Model file for the job. Use its own axes, mm. Face numbers are marked on the shaded views. Give positions to 0.01 mm unless a question says otherwise; leave off trailing zeros. Write each loop counter-clockwise with the first axis right and the second up, starting at its lowest first coordinate (ties: lowest second). Pieces come first, ordered by that corner, then holes.
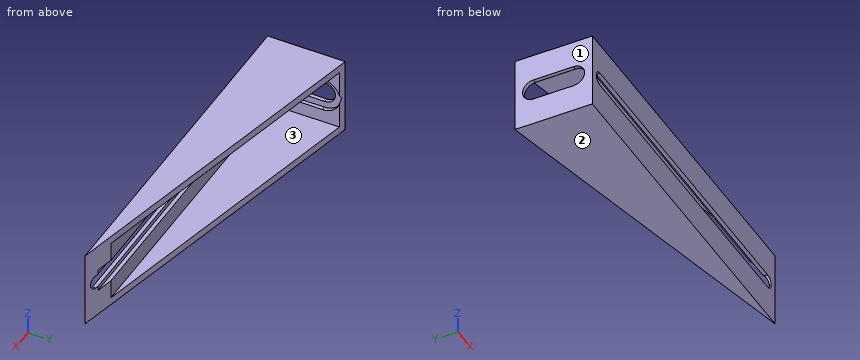
```python
from build123d import *

# Parameters (mm, degrees)
PAD_DEPTH            = 20
SKETCH001_W          = 88
SKETCH001_H          = 16
POCKET_DEPTH         = 18.001
POCKET001_DEPTH      = 2.001
POCKET002_DEPTH      = 1
POCKET002_DEPTH_BACK = -5
POCKET003_DEPTH      = 2.001
POCKET004_DEPTH      = 1


with BuildPart() as part:
    # Sketch → Pad (new body)
    with BuildSketch(Plane.XY):
        Polygon((0, 0), (0, 20), (90, 0), align=None)
    extrude(amount=PAD_DEPTH)

    # Sketch001 → Pocket (cut, through all)
    with BuildSketch(Plane.XZ.offset(-2)):
        with Locations((46, 10)):
            Rectangle(SKETCH001_W, SKETCH001_H)
    extrude(amount=-POCKET_DEPTH, mode=Mode.SUBTRACT)

    # Sketch002 (on Face9 of Pocket) → Pocket001 (cut, through all)
    with BuildSketch(Plane.YZ.offset(2)):
        with BuildLine():
            ThreePointArc((4.8, 12.8), (2, 10), (4.8, 7.2))
            Line((4.8, 7.2), (15.2, 7.2))
            ThreePointArc((15.2, 7.2), (18, 10), (15.2, 12.8))
            Line((4.8, 12.8), (15.2, 12.8))
        make_face()
    extrude(amount=-POCKET001_DEPTH, mode=Mode.SUBTRACT)

    # Sketch003 (on Face13 of Pocket001) → Pocket002 (cut, two sides)
    with BuildSketch(Plane.YZ.offset(2)) as pocket002_sk:
        with BuildLine():
            ThreePointArc((15.2, 5.5), (19.7, 10), (15.2, 14.5))
            Line((4.8, 14.5), (15.2, 14.5))
            ThreePointArc((4.8, 14.5), (3.317186, 14.248678), (2, 13.522783))
            Line((2, 13.522783), (2, 6.477217))
            ThreePointArc((2, 6.477217), (3.317186, 5.751322), (4.8, 5.5))
            Line((4.8, 5.5), (15.2, 5.5))
        make_face()
    extrude(amount=-POCKET002_DEPTH, mode=Mode.SUBTRACT)
    extrude(pocket002_sk.sketch, amount=-POCKET002_DEPTH_BACK, mode=Mode.SUBTRACT)

    # Sketch004 (on Face20 of Pocket002) → Pocket003 (cut, through all)
    with BuildSketch(Plane(origin=(0, 2, 0), x_dir=(-1, 0, 0), z_dir=(0, 1, 0))):
        with BuildLine():
            ThreePointArc((-86.2, 11.8), (-88, 10), (-86.2, 8.2))
            Line((-86.2, 8.2), (-3.8, 8.2))
            ThreePointArc((-3.8, 8.2), (-2, 10), (-3.8, 11.8))
            Line((-86.2, 11.8), (-3.8, 11.8))
        make_face()
    extrude(amount=-POCKET003_DEPTH, mode=Mode.SUBTRACT)

    # Sketch005 (on Face15 of Pocket003) → Pocket004 (cut)
    with BuildSketch(Plane(origin=(0, 2, 0), x_dir=(-1, 0, 0), z_dir=(0, 1, 0))):
        with BuildLine():
            ThreePointArc((-86.2, 13), (-89.2, 10), (-86.2, 7))
            Line((-86.2, 7), (-3.8, 7))
            ThreePointArc((-3.8, 7), (-2.851317, 7.15395), (-2, 7.6))
            Line((-2, 12.4), (-2, 7.6))
            ThreePointArc((-2, 12.4), (-2.851317, 12.84605), (-3.8, 13))
            Line((-86.2, 13), (-3.8, 13))
        make_face()
    extrude(amount=-POCKET004_DEPTH, mode=Mode.SUBTRACT)


solid = part.part
```
1. Slice it at C-C, the plane z = 3.5. Write the cut outline in (x, y).
Calculated:
outline: (0, 0) - (90, 0) - (81, 2) - (2, 2) - (2, 19.56) - (0, 20) - close
2. Slice it at B-B, the plane x = 54. Write the cut outline in (y, z), and give its area (3 significant figures).
Calculated:
outline: (0, 0) - (8, 0) - (8, 2) - (2, 2) - (2, 7) - (1, 7) - (1, 8.2) - (0, 8.2) - close; (0, 11.8) - (1, 11.8) - (1, 13) - (2, 13) - (2, 18) - (8, 18) - (8, 20) - (0, 20) - close
area: 54.4 mm2
3. Probe probe 1 along Z at (x, y) = (37.5, 3.5); probe 2 along X at (y, z) = (15.25, 17); probe 3 along X at (y, z) = (14.25, 13.25). List the from-to ranges inside material, lowest first.
Calculated:
probe 1: z = 0 to 2, 18 to 20
probe 2: x = 0 to 2
probe 3: x = 0 to 1
4. Slice it at A-A, the plane y = 13.5. Write the cut outline in (x, z), and give its area (3 significant figures).
Calculated:
outline: (0, 0) - (29.25, 0) - (29.25, 2) - (2, 2) - (2, 5.5) - (1, 5.5) - (1, 7.2) - (0, 7.2) - close; (0, 12.8) - (1, 12.8) - (1, 14.5) - (2, 14.5) - (2, 18) - (29.25, 18) - (29.25, 20) - (0, 20) - close
area: 134 mm2
5. Pull direction Z, two halves, no side cores. Call the marked faces 1, 2 and 3: +Z half, -Z half, draft (parallel to the pull), parting line (faces both ways), or undercut.
Calculated:
face 1: draft
face 2: -Z half
face 3: undercut
6. Pin check, flat tips, straight feed: P1, Ø5.5, axis at x = 56, y = 9.5, coming from the +Z side; P2, Ø2, axis at y = 12, z = 14.5, coming from the +X side; P3, Ø2.5, axis at x = 51.5, z = 11.5, coming from the +Y side; P4, Ø3.5, axis at x = 54, z = 8.5, coming from the +Y side. Stop position of each tip, or through.
Calculated:
P1: stops at z = 20
P2: stops at x = 2
P3: stops at y = 1
P4: stops at y = 2
